Design review of the part built by this model. Coordinates are the model's own, in mm. A direction names the side the tool comes from. Coordinates: 2 decimals unless noted, no trailing zeros. Loops run counter-clockwise (first coordinate to the right, second up) from the corner with the lowest first, then second, coordinate; pieces in that order, holes last. Notation, with made-up numbers: (-31, 15.5) - (16, 15.5) arc R28 ccw to (16, 54.5) - close; hole circle Ø5 at (-7, -31.5). An arc over 180 degrees is marked (long way). Use one line per item in the form item = value. Start each with the question number.
(1) Clearance check with flat-ended pins moving along their axes: pin 1 Ø1.6 at (x, y) = (-11.5, 0) entering from -Z (3 decimals); pin 2 Ø0.7 at (y, z) = (0.5, 3.5) entering from -X; pin 3 Ø1 at (x, z) = (-5, 8) entering from +Y; pin 4 Ø3.5 at (x, y) = (7, 6) entering from +Z. State where each tip first meets the part, or that it passes through.
(2) The part is to be moulded in two halves that separate along Y. For faces 1 (the face through (0, -2.9, 8)), 2 (the face through (-11, -3.325, 3)), 3 (the face through (15, 0, 3)), 4 (the face through (10, -2, 3)), say which applies: pulls with the +Y half, pulls with the -Y half, needs draft (parallel to the pull), parting line crosses it, or undercut.
(3) For L1, parallel to X at y = 0, z = 7 (3 decimals); L2, parallel to Y at x = -11.5, z = 1.5 (3 decimals); L3, parallel to Z at x = -8.5, y = 2.25, list the stretches that pass through material, from the lowest coordinate up.
(4) Add section A-A (x = -11.5). State the section outline as (y, z) points (3 decimals).
(5) Add section C-C (y = 0). State the section outline as (x, z) points (3 decimals), plus the area to 3 significant figures.
(6) Add section B-B (z = 4.75). State the section outline as (x, y) points (3 decimals), plus the area to 3 significant figures.
(7) Add section D-D (x = 2.5). State the section outline as (y, z) points, plus the area to 3 significant figures.
(8) Tool access review of faces 5 (the face through (5, 0, 1)), 6 (the face through (0, -6, 7)), 7 (the face through (-15, 0, 5)), 8 (the face through (-11, 3.325, 3)): name each direction out of +Z, -Z, +X, -X, +Y, -Y from which nothing blocks a thin tool from reaching the whole face with its end or side.
```python
from build123d import *

# Parameters (mm, degrees)
F0_W     = 30
F0_H     = 2.9
F0_H_2   = 7.1
F1_DEPTH = 7
F2_DEPTH = 9
F3_R     = 1.75
F4_DEPTH = 10
F3_R_2   = 4
F5_DEPTH = 3
F7_START = -8
F6_W     = 6.65
F6_H     = 2.42
F7_DEPTH = 7
F8_R     = 1.325
F9_DEPTH = 25


with BuildPart() as f1:
    # F0 (on Top) → F1 (new body)
    with BuildSketch(Plane.XY):
        with Locations((0, -1.45)):
            Rectangle(F0_W, F0_H)
        with Locations((0, -6.45)):
            Rectangle(F0_W, F0_H_2)
        with Locations((0, 6.45)):
            Rectangle(F0_W, F0_H_2)
        with Locations((0, 1.45)):
            Rectangle(F0_W, F0_H)
    extrude(amount=F1_DEPTH)

    # F0 (on Top) → F2 (join)
    with BuildSketch(Plane.XY):
        with Locations((0, -1.45)):
            Rectangle(F0_W, F0_H)
        with Locations((0, 1.45)):
            Rectangle(F0_W, F0_H)
    extrude(amount=F2_DEPTH)

    # F3 (on Top) → F4 (cut)
    with BuildSketch(Plane.XY):
        with Locations((9, 0)):
            Circle(F3_R)
    extrude(amount=F4_DEPTH, mode=Mode.SUBTRACT)

    # F3 (on Top) → F5 (cut)
    with BuildSketch(Plane.XY):
        with Locations((9, 0)):
            Circle(F3_R_2)
        with Locations((9, 0)):
            Circle(F3_R, mode=Mode.SUBTRACT)
    extrude(amount=F5_DEPTH, mode=Mode.SUBTRACT)

    # F6 (on Right) → F7 (cut)
    with BuildSketch(Plane.YZ.offset(F7_START)):
        with Locations((0, 3.21)):
            Rectangle(F6_W, F6_H)
    extrude(amount=-F7_DEPTH, mode=Mode.SUBTRACT)

    # F8 (on Top) → F9 (cut)
    with BuildSketch(Plane.XY):
        with Locations((-11.5, 0)):
            Circle(F8_R)
    extrude(amount=F9_DEPTH, mode=Mode.SUBTRACT)


solid = f1.part
```
Computed values:
q1.pin_1 = through
q1.pin_2 = -8
q1.pin_3 = 2.9
q1.pin_4 = 7
q2.face_1 = pulls with the -Y half
q2.face_2 = undercut
q2.face_3 = needs draft
q2.face_4 = undercut
q3.L1 = -15 to -12.825, -10.175 to 7.25, 10.75 to 15
q3.L2 = -10 to -1.325, 1.325 to 10
q3.L3 = 0 to 2, 4.42 to 9
q4.outline = (-10, 0) - (-1.325, 0) - (-1.325, 2) - (-3.325, 2) - (-3.325, 4.42) - (-1.325, 4.42) - (-1.325, 9) - (-2.9, 9) - (-2.9, 7) - (-10, 7) - close; (1.325, 0) - (10, 0) - (10, 7) - (2.9, 7) - (2.9, 9) - (1.325, 9) - (1.325, 4.42) - (3.325, 4.42) - (3.325, 2) - (1.325, 2) - close
q5.outline = (-15, 0) - (-12.825, 0) - (-12.825, 2) - (-15, 2) - close; (-15, 4.42) - (-12.825, 4.42) - (-12.825, 9) - (-15, 9) - close; (-10.175, 0) - (5, 0) - (5, 3) - (7.25, 3) - (7.25, 9) - (-10.175, 9) - (-10.175, 4.42) - (-8, 4.42) - (-8, 2) - (-10.175, 2) - close; (10.75, 3) - (13, 3) - (13, 0) - (15, 0) - (15, 9) - (10.75, 9) - close
q5.area = 191 mm^2
q6.outline = (-15, -10) - (15, -10) - (15, 10) - (-15, 10) - close; hole circle Ø2.65 at (-11.5, 0); hole circle Ø3.5 at (9, 0)
q6.area = 585 mm^2
q7.outline = (-10, 0) - (10, 0) - (10, 7) - (2.9, 7) - (2.9, 9) - (-2.9, 9) - (-2.9, 7) - (-10, 7) - close
q7.area = 152 mm^2
q8.face_5 = -Z
q8.face_6 = +Z, +X, -X, -Y
q8.face_7 = +Z, -Z, -X, +Y, -Y
q8.face_8 = -X
